Part model, mm, in its own coordinate system. A direction names the side the tool comes from. Coordinates: 2 decimals unless noted, no trailing zeros. Loops run counter-clockwise (first coordinate to the right, second up) from the corner with the lowest first, then second, coordinate; pieces in that order, holes last.
```python
from build123d import *

# Parameters (mm, degrees)
SKETCH_W     = 30
SKETCH_H     = 40
PAD_DEPTH    = 15
SKETCH001_R  = 10
POCKET_DEPTH = 12
FILLET_R     = 2
FILLET001_R  = 8
FILLET002_R  = 10


with BuildPart() as part:
    # Sketch → Pad (new body)
    with BuildSketch(Plane.XY):
        Rectangle(SKETCH_W, SKETCH_H)
    extrude(amount=PAD_DEPTH)

    # Sketch001 (on Face5 of Pad) → Pocket (cut)
    with BuildSketch(Plane(origin=(0, 0, 0), x_dir=(1, 0, 0), z_dir=(0, 0, -1))):
        Circle(SKETCH001_R)
    extrude(amount=-POCKET_DEPTH, mode=Mode.SUBTRACT)

    # Fillet
    fillet_edges = [part.edges().sort_by_distance(p)[0] for p in [
        (-10, 0, 12),
    ]]
    fillet(fillet_edges, radius=FILLET_R)

    # Fillet001
    fillet001_edges = [part.edges().sort_by_distance(p)[0] for p in [
        (-15, 20, 7.5),
        (-15, -20, 7.5),
        (15, -20, 7.5),
        (15, 20, 7.5),
    ]]
    fillet(fillet001_edges, radius=FILLET001_R)

    # Fillet002
    fillet002_edges = [part.edges().sort_by_distance(p)[0] for p in [
        (0, 20, 15),
        (12.656854, 17.656854, 15),
        (-12.656854, 17.656854, 15),
        (15, 0, 15),
        (-15, 0, 15),
        (12.656854, -17.656854, 15),
        (-12.656854, -17.656854, 15),
        (0, -20, 15),
    ]]
    fillet(fillet002_edges, radius=FILLET002_R)


solid = part.part
```
Q1. Saw through at C-C (x = 0). List the corners of the cut face in (y, z), plus the area to 3 significant figures.
Q2. Saw through at B-B (y = 0). List the corners of the cut face in (x, z).
Q3. Saw through at A-A (z = 4.5). List the corners of the cut face in (x, y), plus the area to 3 significant figures.
Q4. Tool access for faces 1 (the flat face through (0, -20, 2)), 2 (the cylindrical face through (-2.17, 9.76, 4.93)): list every direction of +Z, -Z, +X, -X, +Y, -Y with a clear straight run to the whole face (end or side of a thin tool).
Q5. Drop flat-ended pins along their axis: P1, Ø1, axis at y = -7.5, z = 6, coming from the +X side; P2, Ø8, axis at x = 4, y = 2, coming from the -Z side; P3, Ø1.5, axis at x = -8, z = 11.5, coming from the -Y side. Give the stop position or say it passes through.
Q6. Mould opens along X. For faces 3 (the flat face through (0, 0, 15)), 4 (the flat face through (0, 0, 12)), 5 (the cylindrical face through (12.15, -0.17, 11.99)) say: released by +X, released by -X, zero draft, split by the parting line, or undercut.
Q7. Probe line 1 (Y direction, x = 0, z = 3.5); line 2 (X direction, y = 0, z = 3.5); line 3 (Z direction, x = 4, y = -5.5). List the from-to ranges inside material, lowest first.
Checked values:
1. outline: (-20, 0) - (-10, 0) - (-10, 10) arc R2 cw to (-8, 12) - (8, 12) arc R2 cw to (10, 10) - (10, 0) - (20, 0) - (20, 5) arc R10 ccw to (10, 15) - (-10, 15) arc R10 ccw to (-20, 5) - close
1. area: 319 mm2
2. outline: (-15, 0) - (-10, 0) - (-10, 10) arc R2 cw to (-8, 12) - (8, 12) arc R2 cw to (10, 10) - (10, 0) - (15, 0) - (15, 5) arc R10 ccw to (5, 15) - (-5, 15) arc R10 ccw to (-15, 5) - close
3. outline: (-15, -12) arc R8 ccw to (-7, -20) - (7, -20) arc R8 ccw to (15, -12) - (15, 12) arc R8 ccw to (7, 20) - (-7, 20) arc R8 ccw to (-15, 12) - close; hole circle Ø20 at (0, 0)
3. area: 831 mm2
4. face 1: +Z, -Z, +X, -X, -Y
4. face 2: -Z
5. P1: stops at x = 14.99
5. P2: stops at z = 11.94
5. P3: stops at y = -17.96
6. face 3: zero draft
6. face 4: undercut
6. face 5: released by +X
7. line 1: y = -20 to -10, 10 to 20
7. line 2: x = -15 to -10, 10 to 15
7. line 3: z = 12 to 15
